from build123d import *

# Parameters (mm, degrees)
F1_DEPTH = 10
F3_D     = 4


with BuildPart() as f1:
    # F0 (on Top) → F1 (new body)
    with BuildSketch(Plane.XY):
        Polygon((0, -3), (0, 0), (-10, 0), (-10, -10), (-3, -10), (-3, -14), (-10, -14), (-10, -24), (0, -24), (0, -21), (-7, -21), (-7, -17), (0, -17), (0, -7), (-7, -7), (-7, -3), align=None)
    extrude(amount=F1_DEPTH)

    # F3 (through all)
    with Locations(Plane(origin=(0, 0, 0), x_dir=(-1, 0, 0), z_dir=(0, 1, 0))):
        with Locations((5, 5)):
            Hole(F3_D / 2)


solid = f1.part
Model file for the job. Use its own axes, mm. A direction names the side the tool comes from. Give positions to 0.01 mm unless a question says otherwise; leave off trailing zeros. Order: outer loops, then holes, each group sorted by start corner. A loop starts at its lowest first (then second) coordinate and runs counter-clockwise, first axis right, second up. Notation, with made-up numbers: (84, -10.5) -> (134, -10.5) arc R31 cw to (134, 15.5) -> close; hole circle Ø3 at (33.5, 63.5). An arc over 180 degrees is marked (long way). Use CSV: the item, a comma, the result in double quotes.
1. Mould opens along Y. For faces 1 (the flat face through (0, -12, 5)), 2 (the flat face through (-7.2, -14, 4.9)), 3 (the flat face through (-2.8, -24, 4.9)) say: +Y half, -Y half, draft (parallel to the pull), parting line (faces both ways), or undercut.
Outcome:
face 1,"draft"
face 2,"undercut"
face 3,"-Y half"
2. Band-saw the part on A-A, the plane x = -5. Count the separate pieces of the cut face and the enclosed holes in it, then the cut area to 3 significant figures.
Outcome:
separate pieces,"8"
enclosed holes,"0"
area,"72.0 mm²"
3. Drill centre lines: line 1 along Y through (x, z) = (-4.5, 1.5); line 2 along X through (y, z) = (-1.55, 5); line 3 along Z through (x, y) = (-5, -22.35). Where is each one in solid material? Low to high. Write a range as from..to.
Outcome:
line 1,"-24..-21, -17..-14, -10..-7, -3..0"
line 2,"-10..-7, -3..0"
line 3,"0..3, 7..10"
4. Band-saw the part on C-C, the plane x = -8. Give the cut face in (y, z), then the cut area to 3 significant figures.
Outcome:
outline,"(-24, 0) -> (-14, 0) -> (-14, 10) -> (-24, 10) -> close; (-10, 0) -> (0, 0) -> (0, 10) -> (-10, 10) -> close"
area,"200 mm²"
5. Band-saw the part on D-D, the plane y = -16.5. Give the cut face in (x, z).
Outcome:
outline,"(-10, 0) -> (0, 0) -> (0, 10) -> (-10, 10) -> close; hole circle Ø4 at (-5, 5)"
6. Drop a flat-ended pin along its axis: pin 1 (1.2 mm diameter, centred on y = -12.5, z = 7, fed in from -X). Give the stop position or say it passes through.
Outcome:
pin 1,"x = -3"
7. 3-axis set-ups, long thin cutter, end or side, ignore diameter. For faces 4 (the flat face through (-2.8, -17, 4.9)), 5 (the cylindrical face through (-7, -2, 5)): which of +Z, -Z, +X, -X, +Y, -Y reach the whole face in a straight line?
Outcome:
face 4,"+Z, -Z, +X"
face 5,"+Y, -Y"
